Build history of the part. All positions in model axes, mm. A direction names the side the tool comes from. Round coordinates to 2 decimals unless told otherwise and drop trailing zeros. Loops run counter-clockwise (first coordinate to the right, second up) from the corner with the lowest first, then second, coordinate; pieces in that order, holes last. Notation, with made-up numbers: (66.25, 50) -> (90.25, 50) arc R16 cw to (90.25, 61) -> close; hole circle Ø9 at (-12, 77.5). An arc over 180 degrees is marked (long way). Put each result on its own line as item: value. Start each with the question number.
Item 1: Tool access for faces 1 (the flat face through (10, 7, -4.6)), 2 (the flat face through (10, 7, 5.4)), 3 (the flat face through (-12.75, 7, -5)): list every direction of +Z, -Z, +X, -X, +Y, -Y with a clear straight run to the whole face (end or side of a thin tool).
Item 2: Flat gauge pins, fed straight in: pin 1 Ø0.9 at (y, z) = (6.5, 5) entering from +X; pin 2 Ø1 at (x, y) = (-9.5, 7) entering from -Z; pin 3 Ø2 at (x, y) = (-11, 7.5) entering from +Z. Where does each tip first touch, or does it go through?
Item 3: Pull direction Z, two halves, no side cores. Call faces 4 (the cylindrical face through (0.27, 2.27, 1.45)), 5 (the flat face through (20.5, 3, 0)), 6 (the flat face through (10, 7, 4.6)), 7 (the flat face through (-10, 7, -5.4)): +Z half, -Z half, draft (parallel to the pull), parting line (faces both ways), or undercut.
Item 4: Cut at A-A, the plane x = 9. List the corners of the cut face in (y, z).
Item 5: Drill centre lines: probe 1 along X at (y, z) = (3.25, 1.5); probe 2 along X at (y, z) = (1, -2); probe 3 along Z at (x, y) = (15, 5.75). Where is each one in solid material? Low to high. Write a range as [from, to].
Item 6: Cut at C-C, the plane z = 3. List the corners of the cut face in (x, y).
Item 7: Cut at D-D, the plane y = 3.25. List the corners of the cut face in (x, z).
Item 8: Cut at B-B, the plane y = 6.5. List the corners of the cut face in (x, z).
```python
from build123d import *

# Parameters (mm, degrees)
BOSS_EXTRUDE2_DEPTH = 20.5
SKETCH4_W           = 5
SKETCH4_H           = 8.500741967
CUT_EXTRUDE1_DEPTH  = 45
BOSS_EXTRUDE4_DEPTH = 1
SKETCH3_W           = 5
SKETCH3_H           = 0.8
BOSS_EXTRUDE5_DEPTH = 2


with BuildPart() as part:
    # Sketch2 → Boss-Extrude2 (new body, symmetric)
    with BuildSketch(Plane(origin=(0, 0, 0), x_dir=(0, 0, -1), z_dir=(1, 0, 0))):
        with BuildLine():
            Line((-6, 6), (-4, 6))
            ThreePointArc((-4, 6), (0, 2), (4, 6))
            Line((4, 6), (6, 6))
            Line((6, 6), (6, 0))
            Line((6, 0), (-6, 0))
            Line((-6, 0), (-6, 6))
        make_face()
    extrude(amount=BOSS_EXTRUDE2_DEPTH, both=True)

    # Sketch4 → Cut-Extrude1 (cut)
    with BuildSketch(Plane.XZ):
        with Locations((0, -4.250370983)):
            Rectangle(SKETCH4_W, SKETCH4_H)
    extrude(amount=-CUT_EXTRUDE1_DEPTH, mode=Mode.SUBTRACT)

    # Sketch5 → Boss-Extrude4 (add)
    with BuildSketch(Plane.ZY.offset(20.5)):
        with BuildLine():
            Line((-4, 6), (-1, 6))
            ThreePointArc((-1, 6), (0, 5), (1, 6))
            Line((1, 6), (4, 6))
            ThreePointArc((4, 6), (0, 2), (-4, 6))
        make_face()
    boss_extrude4 = extrude(amount=-BOSS_EXTRUDE4_DEPTH)

    # Mirror1: Boss-Extrude4 across plane
    add(boss_extrude4.mirror(Plane(origin=(0, 0, 0), x_dir=(0, 0, 1), z_dir=(1, 0, 0))))

    # Sketch3 → Boss-Extrude5 (add)
    with BuildSketch(Plane(origin=(0, 6, 0), x_dir=(1, 0, 0), z_dir=(0, 1, 0))):
        with Locations((-10.25, 5)):
            Rectangle(SKETCH3_W, SKETCH3_H)
        with Locations((-10.25, -5)):
            Rectangle(SKETCH3_W, SKETCH3_H)
        with Locations((10.25, -5)):
            Rectangle(SKETCH3_W, SKETCH3_H)
        with Locations((10.25, 5)):
            Rectangle(SKETCH3_W, SKETCH3_H)
    extrude(amount=BOSS_EXTRUDE5_DEPTH)


solid = part.part
```
Reply:
1. face 1: +X, -X, +Y
1. face 2: +Z, +X, -X, +Y
1. face 3: +Z, -Z, -X, +Y
2. pin 1: stops at x = 12.75
2. pin 2: stops at z = -5.4
2. pin 3: stops at z = 5.4
3. face 4: undercut
3. face 5: draft
3. face 6: undercut
3. face 7: -Z half
4. outline: (0, -6) -> (6, -6) -> (6, -5.4) -> (8, -5.4) -> (8, -4.6) -> (6, -4.6) -> (6, -4) arc R4 cw to (6, 4) -> (6, 4.6) -> (8, 4.6) -> (8, 5.4) -> (6, 5.4) -> (6, 6) -> (0, 6) -> close
5. probe 1: x = [-20.5, -19.5], [19.5, 20.5]
5. probe 2: x = [-20.5, -2.5], [2.5, 20.5]
5. probe 3: z = [-6, -3.99], [3.99, 6]
6. outline: (-20.5, 0) -> (20.5, 0) -> (20.5, 6) -> (19.5, 6) -> (19.5, 3.35) -> (-19.5, 3.35) -> (-19.5, 6) -> (-20.5, 6) -> close
7. outline: (-20.5, -6) -> (-2.5, -6) -> (-2.5, -2.9) -> (-19.5, -2.9) -> (-19.5, 2.9) -> (19.5, 2.9) -> (19.5, -2.9) -> (2.5, -2.9) -> (2.5, -6) -> (20.5, -6) -> (20.5, 6) -> (-20.5, 6) -> close
8. outline: (-12.75, -5.4) -> (-7.75, -5.4) -> (-7.75, -4.6) -> (-12.75, -4.6) -> close; (-12.75, 4.6) -> (-7.75, 4.6) -> (-7.75, 5.4) -> (-12.75, 5.4) -> close; (7.75, -5.4) -> (12.75, -5.4) -> (12.75, -4.6) -> (7.75, -4.6) -> close; (7.75, 4.6) -> (12.75, 4.6) -> (12.75, 5.4) -> (7.75, 5.4) -> close
